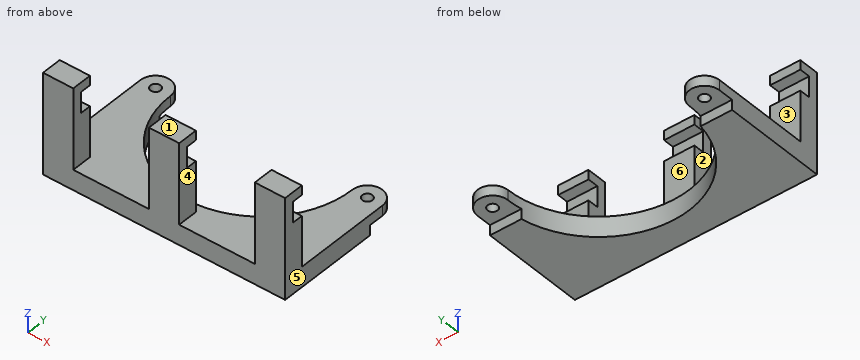
from build123d import *

# Parameters (mm, degrees)
F0_R     = 2.5
F1_DEPTH = 10
F3_DEPTH = 5
F4_W     = 15
F4_H     = 10
F5_DEPTH = 40
F6_W     = 5.3
F6_H     = 10.3
F7_DEPTH = 120.001


with BuildPart() as f1:
    # F0 (on Top) → F1 (new body)
    with BuildSketch(Plane.XY):
        with BuildLine():
            ThreePointArc((105, 7.5), (60, -37.5), (15, 7.5))
            ThreePointArc((15, 7.5), (7.5, 15), (0, 7.5))
            Line((0, 7.5), (0, -51))
            Line((0, -51), (120, -51))
            Line((120, -51), (120, 7.5))
            ThreePointArc((120, 7.5), (112.5, 15), (105, 7.5))
        make_face()
        with Locations((7.5, 7.5)):
            Circle(F0_R, mode=Mode.SUBTRACT)
        with Locations((112.5, 7.5)):
            Circle(F0_R, mode=Mode.SUBTRACT)
    extrude(amount=F1_DEPTH)

    # F2 (on face) → F3 (cut)
    with BuildSketch(Plane(origin=(0, 0, 0), x_dir=(1, 0, 0), z_dir=(0, 0, -1))):
        with BuildLine():
            ThreePointArc((0, -7.5), (7.5, -15), (15, -7.5))
            ThreePointArc((15, -7.5), (15.157626, -3.736818), (15.629402, 0))
            Line((15.629402, 0), (0, 0))
            Line((0, 0), (0, -7.5))
        make_face()
        with BuildLine():
            ThreePointArc((15.629402, 0), (15.157626, -3.736818), (15, -7.5))
            ThreePointArc((15, -7.5), (60, -52.5), (105, -7.5))
            ThreePointArc((105, -7.5), (112.5, -15), (120, -7.5))
            Line((120, -7.5), (120, 0))
            Line((120, 0), (104.370598, 0))
            ThreePointArc((104.370598, 0), (60, 37.5), (15.629402, 0))
        make_face()
    extrude(amount=-F3_DEPTH, mode=Mode.SUBTRACT)

    # F4 (on face) → F5 (join)
    with BuildSketch(Plane.XY.offset(10)):
        with Locations((7.5, -46)):
            Rectangle(F4_W, F4_H)
        with Locations((112.5, -46)):
            Rectangle(F4_W, F4_H)
        with Locations((60, -46)):
            Rectangle(F4_W, F4_H)
    extrude(amount=F5_DEPTH)

    # F6 (on face) → F7 (cut, through all)
    with BuildSketch(Plane(origin=(0, 0, 0), x_dir=(0, -1, 0), z_dir=(-1, 0, 0))):
        with Locations((43.65, 40.15)):
            Rectangle(F6_W, F6_H)
    extrude(amount=-F7_DEPTH, mode=Mode.SUBTRACT)


solid = f1.part
Geometry: final body of the model. Coordinates: model frame, mm. Face numbers are marked on the shaded views. A direction names the side the tool comes from. Round coordinates to 2 decimals unless told otherwise and drop trailing zeros. Loops run counter-clockwise (first coordinate to the right, second up) from the corner with the lowest first, then second, coordinate; pieces in that order, holes last.
Q1. Section A-A on x = 7.5. Return loops of the section in (y, z), plus the area to 3 significant figures.
Q2. Pull-direction query (X, two-part tool) for the marked faces 4, 5 and 6; classes: released by +X, released by -X, zero draft, split by the parting line, or undercut.
Q3. Material intervals for L1, parallel to X at y = -45.5, z = 20; L2, parallel to X at y = 7.5, z = 6.35; L3, parallel to Y at x = 112.5, z = 8.1, sorted ascending.
Q4. Access query for the marked faces 1, 2 and 3. Directions: +Z, -Z, +X, -X, +Y, -Y. A direction counts if a zero-diameter tool reaches every point of the face in a straight line with its end or side. Return the directions, or none.
Q5. Section B-B on z = 29. Return loops of the section in (x, y), plus the area to 3 significant figures.
Q6. Section D-D on x = 60. Return loops of the section in (y, z), plus the area to 3 significant figures.
Q7. Pin query (flat end, axial travel): P1, Ø6, axis at y = -15.5, z = 15, coming from the -X side; P2, Ø6, axis at x = 107, y = -14, coming from the +Z side; P3, Ø1.4, axis at x = 109.5, z = 47.5, coming from the +Y side; P4, Ø1.5, axis at x = 10.5, z = 3, coming from the +Y side. Return the tip coordinate at first contact, or that it passes through.
Q8. Section C-C on y = -12. Return loops of the section in (x, z), plus the area to 3 significant figures.
Evaluation:
1. outline: (-51, 0) - (0, 0) - (0, 5) - (5, 5) - (5, 10) - (-41, 10) - (-41, 35) - (-46.3, 35) - (-46.3, 45.3) - (-41, 45.3) - (-41, 50) - (-51, 50) - close; (10, 5) - (15, 5) - (15, 10) - (10, 10) - close
1. area: 905 mm2
2. face 4: undercut
2. face 5: released by +X
2. face 6: zero draft
3. L1: x = 0 to 15, 52.5 to 67.5, 105 to 120
3. L2: x = 0 to 5, 10 to 15, 105 to 110, 115 to 120
3. L3: y = -51 to 5, 10 to 15
4. face 1: +Z, +X, -X, +Y, -Y
4. face 2: +Z, +Y, -Y
4. face 3: +Z, +X, -X, +Y
5. outline: (0, -51) - (15, -51) - (15, -41) - (0, -41) - close; (52.5, -51) - (67.5, -51) - (67.5, -41) - (52.5, -41) - close; (105, -51) - (120, -51) - (120, -41) - (105, -41) - close
5. area: 450 mm2
6. outline: (-51, 0) - (-37.5, 0) - (-37.5, 10) - (-41, 10) - (-41, 35) - (-46.3, 35) - (-46.3, 45.3) - (-41, 45.3) - (-41, 50) - (-51, 50) - close
6. area: 480 mm2
7. P1: passes through
7. P2: stops at z = 10
7. P3: stops at y = -41
7. P4: stops at y = 0
8. outline: (0, 0) - (19.44, 0) - (19.44, 10) - (0, 10) - close; (100.56, 0) - (120, 0) - (120, 10) - (100.56, 10) - close
8. area: 389 mm2
